Check sheet for the drawn part. Datum: minimum x, y, z corner. Units: mm. Give positions to 0.01 mm unless a question says otherwise; leave off trailing zeros. Order: outer loops, then holes, each group sorted by start corner. A loop starts at its lowest first (then second) coordinate and runs counter-clockwise, first axis right, second up. Notation, with made-up numbers: M -33.5,83.25 L -16.5,83.25 A23 ccw -16.5,93.25 Z; hole C -20,-23.75 d3. An arc over 180 degrees is marked long. Put each result on its own line as item: value. Start each with the question number.
Q1. Section check C-C on x = 834.5. Record the cut outline in (y, z).
Q2. Section check B-B on y = 162. Record the cut outline in (x, z).
Q3. Go/stop test with flat-tipped pins: pin 1 (9.5 mm diameter, centred on x = 885.5, z = 12, fed in from -Y); pin 2 (2 mm diameter, centred on x = 609, y = 240, fed in from -Z); pin 3 (3 mm diameter, centred on y = 301, z = 6.5, fed in from -X). Record where each tip stops, or that it passes through.
Q4. Material ranges on L1, parallel to Y at x = 823.5, z = 13.75; L2, parallel to X at y = 304, z = 5.5; L3, parallel to X at y = 234, z = 15.75, recorded low to high.
Q5. Section check A-A on z = 8.5. Record the cut outline in (x, y).
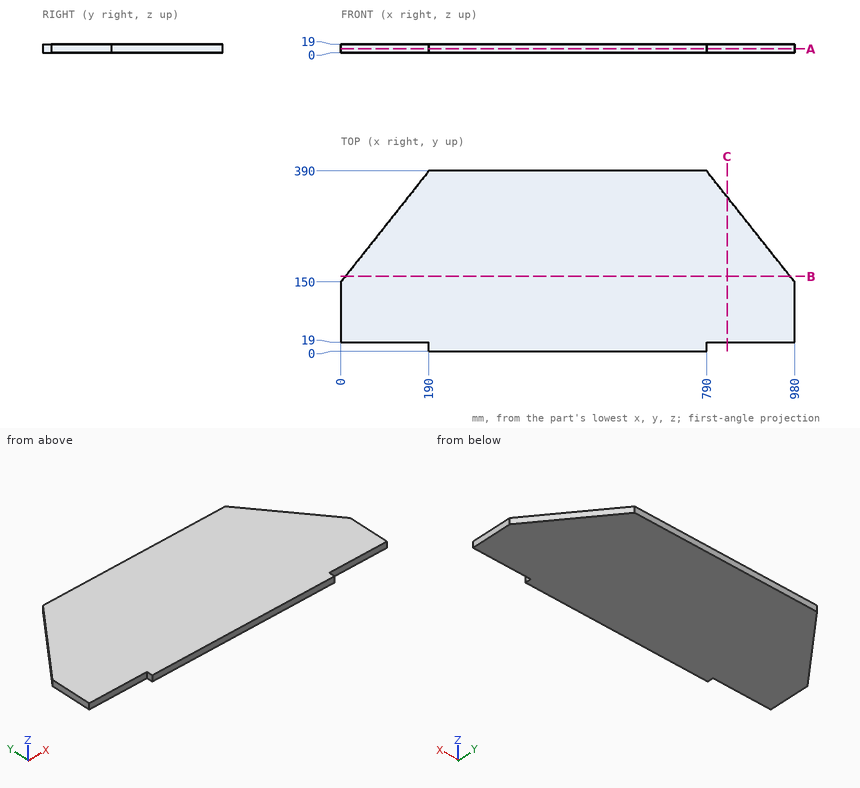
Results found:
1. outline: M 19,0 L 333.79,0 L 333.79,19 L 19,19 Z
2. outline: M 9.5,0 L 970.5,0 L 970.5,19 L 9.5,19 Z
3. pin 1: stops at y = 19
3. pin 2: stops at z = 0
3. pin 3: stops at x = 118.35
4. L1: y = 19 to 347.68
4. L2: x = 121.92 to 858.08
4. L3: x = 66.5 to 913.5
5. outline: M 0,19 L 190,19 L 190,0 L 790,0 L 790,19 L 980,19 L 980,150 L 790,390 L 190,390 L 0,150 Z
